CAD build for the part. Positions are in the model's coordinates, mm. Face numbers are marked on the shaded views. Round coordinates to 2 decimals unless told otherwise and drop trailing zeros. Loops run counter-clockwise (first coordinate to the right, second up) from the corner with the lowest first, then second, coordinate; pieces in that order, holes last.
from build123d import *

# Parameters (mm, degrees)
F1_DEPTH = 5.08
F2_DEPTH = 7.62
F3_D     = 15.24
F4_D     = 12.7


with BuildPart() as f1:
    # F0 (on Top) → F1 (new body)
    with BuildSketch(Plane.XY):
        Polygon((7.62, 25.4), (0, 0), (38.1, 0), (30.48, 25.4), align=None)
        Polygon((27.94, 8.4582), (10.16, 8.4582), (12.69746, 16.9164), (25.40254, 16.9164), align=None, mode=Mode.SUBTRACT)
        Polygon((12.69746, 16.9164), (10.16, 8.4582), (27.94, 8.4582), (25.40254, 16.9164), align=None)
    extrude(amount=F1_DEPTH)

    # F0 (on Top) → F2 (join)
    with BuildSketch(Plane.XY):
        Polygon((12.69746, 16.9164), (10.16, 8.4582), (27.94, 8.4582), (25.40254, 16.9164), align=None)
    extrude(amount=F2_DEPTH)

    # F3 (through all)
    with Locations(Plane(origin=(0, 0, 0), x_dir=(1, 0, 0), z_dir=(0, 0, -1))):
        with Locations((19.05, 2.54)):
            Hole(F3_D / 2)

    # F4 (through all)
    with Locations(Plane(origin=(0, 0, 0), x_dir=(1, 0, 0), z_dir=(0, 0, -1))):
        with Locations((19.05, -27.94)):
            Hole(F4_D / 2)


solid = f1.part
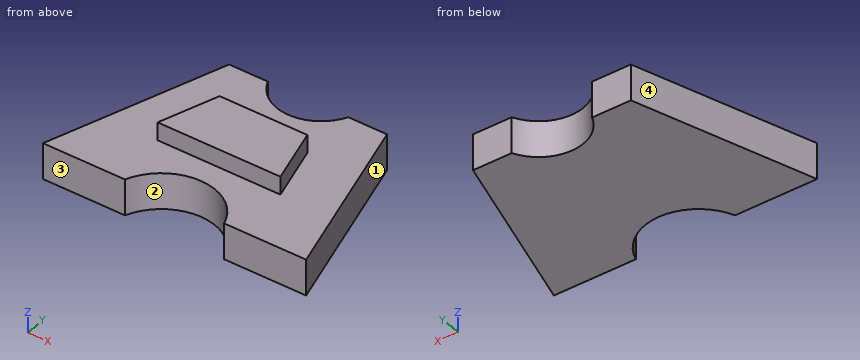
Item 1: Cut at B-B (x = 16). List the corners of the cut face in (y, z).
Verdict:
outline: (4.44, 0) - (22.37, 0) - (22.37, 5.08) - (16.92, 5.08) - (16.92, 7.62) - (8.46, 7.62) - (8.46, 5.08) - (4.44, 5.08) - close
Item 2: Wall check: L1, parallel to Z at x = 13.5, y = 5.5; L2, parallel to Y at x = 16, z = 7.25; L3, parallel to Y at x = 17, z = 1.25. Give the ranges that are in metal, low to high.
Verdict:
L1: z = 0 to 5.08
L2: y = 8.46 to 16.92
L3: y = 4.8 to 21.93
Item 3: Mould opens along X. For the marked faces 1, 2, 3 and 4 say: released by +X, released by -X, zero draft, split by the parting line, or undercut.
Verdict:
face 1: released by +X
face 2: undercut
face 3: zero draft
face 4: released by -X
Item 4: Cut at D-D (z = 5.5). List the corners of the cut face in (x, y).
Verdict:
outline: (10.16, 8.46) - (27.94, 8.46) - (25.4, 16.92) - (12.7, 16.92) - close
Item 5: Flat gauge pins, fed straight in: P1, Ø4, axis at y = 15, z = 3, coming from the -X side; P2, Ø2, axis at x = 12, z = 1.5, coming from the -Y side; P3, Ø0.8, axis at x = 20.5, z = 6.5, coming from the -Y side; P4, Ø3, axis at x = 21, z = 6.5, coming from the +Y side. Where does each tip first touch, or does it go through?
Verdict:
P1: stops at x = 3.9
P2: stops at y = 0
P3: stops at y = 8.46
P4: stops at y = 22.07
Item 6: Cut at C-C (y = 19.5). List the corners of the cut face in (x, z), plus the area to 3 significant figures.
Verdict:
outline: (5.85, 0) - (32.25, 0) - (32.25, 5.08) - (5.85, 5.08) - close
area: 134 mm2
Item 7: Cut at A-A (z = 2). List the corners of the cut face in (x, y).
Verdict:
outline: (0, 0) - (11.87, 0) arc R7.62 cw to (26.23, 0) - (38.1, 0) - (30.48, 25.4) - (24.87, 25.4) arc R6.35 cw to (13.23, 25.4) - (7.62, 25.4) - close
